Model file for the job. Use its own axes, mm. Round coordinates to 2 decimals unless told otherwise and drop trailing zeros. Order: outer loops, then holes, each group sorted by start corner. A loop starts at its lowest first (then second) coordinate and runs counter-clockwise, first axis right, second up. Notation, with made-up numbers: (5.25, 89.25) - (13.25, 89.25) arc R25 cw to (13.25, 121.25) - close; hole circle Ø7 at (66, 1). An arc over 180 degrees is marked (long way). Write item = value, one per line.
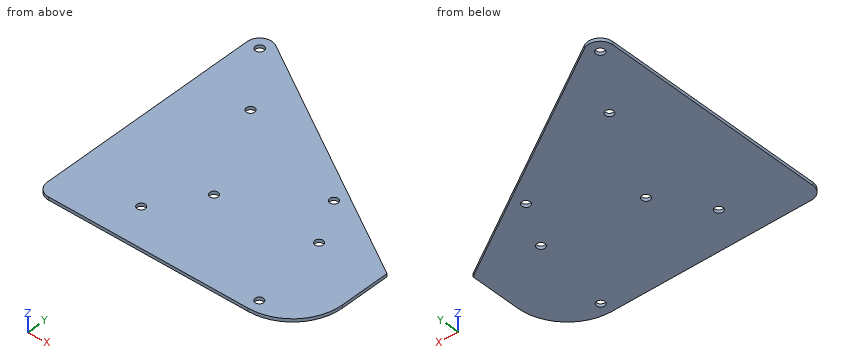
Autodesk Inventor part; units mm, degrees
ref_plane "YZ Plane" through (0, 0, 0) normal (1, 0, 0) x (0, 1, 0)
ref_plane "XZ Plane" through (0, 0, 0) normal (0, 1, 0) x (-1, 0, 0)
ref_plane "XY Plane" through (0, 0, 0) normal (0, 0, 1) x (1, 0, 0)
sketch "Block1" plane through (0, 0, 0) normal (0, 0, 1) x (1, 0, 0)
  circle A0 centre (36.7608, -51.6694) radius 2.0955
  circle A1 centre (30.4108, -10.3944) radius 2.0955
  circle A2 centre (17.7108, 12.3965) radius 2.0955
  circle A3 centre (-18.8017, -15.1569) radius 2.0955
  circle A4 centre (-34.6767, -38.9694) radius 2.0955
  line L0 (-64.8392, -58.0194) -> (36.7608, -58.0194)
  line L1 (62.1608, -7.2194) -> (-61.5382, 68.0552)
  circle A5 centre (-42.6142, 32.4681) radius 2.0955
  circle A6 centre (-64.8392, 62.6306) radius 2.1844
  arc A7 (-61.5382, 68.0552) -> (-71.1892, 62.6306) centre (-64.8392, 62.6306) ccw
  line L2 (-71.1892, -51.6694) -> (-71.1892, 62.6306)
  arc A8 (-71.1892, -51.6694) -> (-64.8392, -58.0194) centre (-64.8392, -51.6694) ccw
  line L3 (62.1608, -32.6194) -> (62.1608, -7.2194)
  arc A9 (36.7608, -58.0194) -> (62.1608, -32.6194) centre (36.7608, -32.6194) ccw
  point P0 (-13.0925, -13.6067)
  point P1 (62.1608, -58.0194)
  dimension "d0" = 12.7
  dimension "d1" = 12.7
  dimension "d2" = 50.8
  dimension "d3" = 25.4
  dimension "d4" = 4.191
  dimension "d5" = 4.191
  dimension "d6" = 4.191
  dimension "d7" = 4.191
  dimension "d8" = 4.191
  dimension "d9" = 4.191
sketch "main" plane through (0, 0, 0) normal (0, 0, 1) x (1, 0, 0)
  circle A0 centre (36.7608, -51.6694) radius 2.0955
  circle A1 centre (30.4108, -10.3944) radius 2.0955
  circle A2 centre (17.7108, 12.3965) radius 2.0955
  circle A3 centre (-18.8017, -15.1569) radius 2.0955
  circle A4 centre (-34.6767, -38.9694) radius 2.0955
  line L0 (-64.8392, -58.0194) -> (36.7608, -58.0194)
  line L1 (62.1608, -7.2194) -> (-61.5382, 68.0552)
  circle A5 centre (-42.6142, 32.4681) radius 2.0955
  circle A6 centre (-64.8392, 62.6306) radius 2.1844
  arc A7 (-61.5382, 68.0552) -> (-71.1892, 62.6306) centre (-64.8392, 62.6306) ccw
  line L2 (-71.1892, -51.6694) -> (-71.1892, 62.6306)
  arc A8 (-71.1892, -51.6694) -> (-64.8392, -58.0194) centre (-64.8392, -51.6694) ccw
  line L3 (62.1608, -32.6194) -> (62.1608, -7.2194)
  arc A9 (36.7608, -58.0194) -> (62.1608, -32.6194) centre (36.7608, -32.6194) ccw
  point P0 (-13.0925, -13.6067)
sketch "Sketch1" plane through (0, 0, 0) normal (0, 0, 1) x (1, 0, 0)
  circle A0 centre (12.7, 0) radius 2.0955
  circle A1 centre (101.6, 0) radius 2.0955
  circle A2 centre (95.25, 41.275) radius 2.0955
  circle A3 centre (82.55, 64.0658) radius 2.0955
  circle A4 centre (46.0375, 36.5125) radius 2.0955
  circle A5 centre (30.1625, 12.7) radius 2.0955
  line L0 (0, -6.35) -> (101.6, -6.35)
  line L1 (127, 44.45) -> (3.301, 119.7246)
  circle A6 centre (22.225, 84.1375) radius 2.0955
  circle A7 centre (0, 114.3) radius 2.1844
  arc A8 (3.301, 119.7246) -> (-6.35, 114.3) centre (0, 114.3) ccw
  line L2 (-6.35, 0) -> (-6.35, 114.3)
  arc A9 (-6.35, 0) -> (0, -6.35) centre (0, 0) ccw
  line L3 (127, 19.05) -> (127, 44.45)
  arc A10 (101.6, -6.35) -> (127, 19.05) centre (101.6, 19.05) ccw
  dimension "d12" = 4.191
extrude "Extrusion1" add sketch "Sketch1" along normal blind 1.5875 contours A0 | A9 L2 A8 L1 L3 A10 L0
equation "\"BendRadius\" = Thickness"
equation "\"BendReliefWidth\" = Thickness"
equation "\"BendReliefDepth\" = 0.5 * Thickness"
equation "\"CornerReliefSize\" = 4 * Thickness"
equation "\"MinimumRemnant\" = 2 * Thickness"
equation "\"TransitionRadius\" = BendRadius"
equation "\"JacobiRadiusSize\" = BendRadius"
equation "\"GapSize\" = Thickness"
properties part number "blocker" material "Acetal Resin, White"
1) Flat gauge pin, fed straight in: pin 1 Ø2.5 at (x, y) = (46.04, 36.51) entering from +Z. Where does the tip first touch, or does it go through?
Conclusion:
pin_1 = through
2) Cut at A-A (x = 95.25). Write the cut outline in (y, z), and give its area (3 significant figures).
Conclusion:
outline = (-6.35, 0) - (39.18, 0) - (39.18, 1.59) - (-6.35, 1.59) - close; (43.37, 0) - (63.77, 0) - (63.77, 1.59) - (43.37, 1.59) - close
area = 105 mm^2
3) Cut at D-D (x = 35.5). Write the cut outline in (y, z), and give its area (3 significant figures).
Conclusion:
outline = (-6.35, 0) - (100.13, 0) - (100.13, 1.59) - (-6.35, 1.59) - close
area = 169 mm^2
4) Wall check: line 1 along Y through (x, z) = (0, 1.25); line 2 along X through (y, z) = (41.5, 0.3); line 3 along Y through (x, z) = (82.55, 0.8). Give the ranges that are in metal, low to high.
Conclusion:
line_1 = -6.35 to 112.12, 116.48 to 120.65
line_2 = -6.35 to 93.17, 97.33 to 127
line_3 = -6.35 to 61.97, 66.16 to 71.5
5) Cut at C-C (y = 12.7). Write the cut outline in (x, z).
Conclusion:
outline = (-6.35, 0) - (28.07, 0) - (28.07, 1.59) - (-6.35, 1.59) - close; (32.26, 0) - (126.19, 0) - (126.19, 1.59) - (32.26, 1.59) - close
6) Cut at B-B (z = 1.1). Give the number of separate pieces and of enclosed holes in the cut face, and give its area (3 significant figures).
Conclusion:
separate_pieces = 1
enclosed_holes = 7
area = 11,900 mm^2
